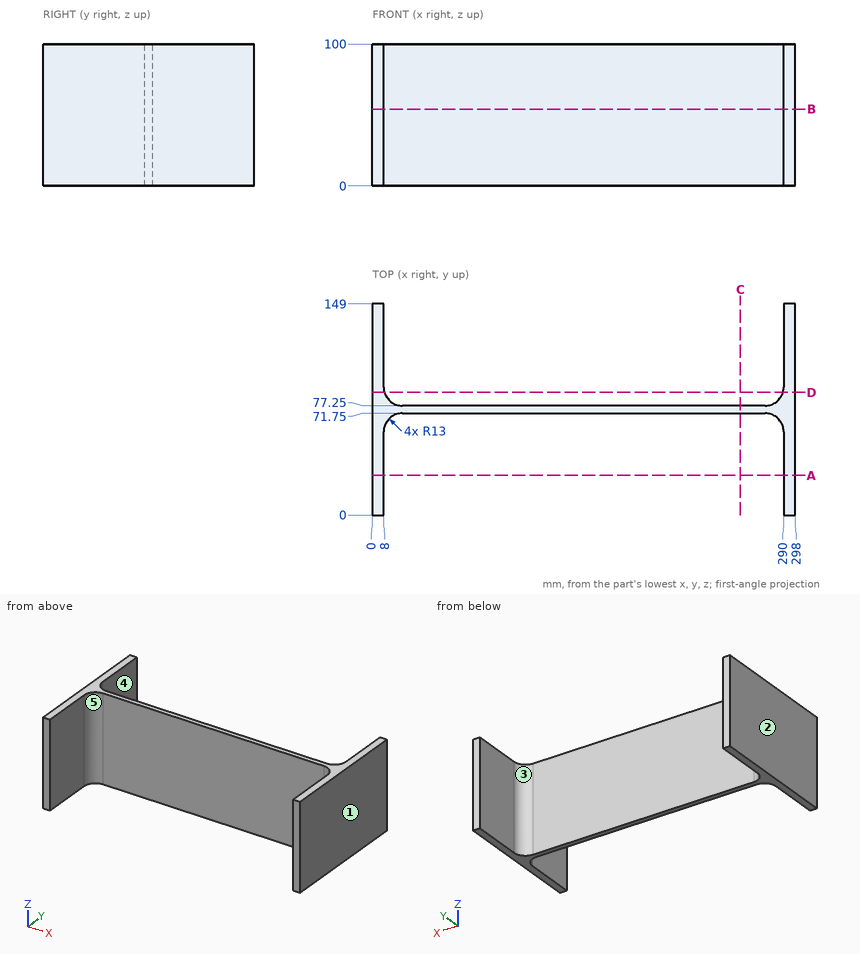
Can you work these out from the drawing? Everything is in mm from the part's minimum corner. A direction names the side the tool comes from. Give positions to 0.01 mm unless a question says otherwise; leave off trailing zeros. Order: outer loops, then holes, each group sorted by start corner. A loop starts at its lowest first (then second) coordinate and runs counter-clockwise, first axis right, second up. Notation, with made-up numbers: M 60.5,8.25 L 67.5,8.25 A17 ccw 67.5,30.25 Z; hole C 27,-3.75 d9. An arc over 180 degrees is marked long. Use a Markdown table: item, result. Add a question column.
Item 1: Suppose I cut it at A-A (y = 28). List the corners of the cut face in (x, z) for me.
Item 2: If I drill on L1, parallel to X at y = 108.5, z = 55.5; L2, parallel to Y at x = 226, z = 21; L3, parallel to X at y = 62, z = 65, over which ranges is the centre line in solid material (lowest first)? Write a range as [from, to].
Item 3: For the marked faces 4 and 5, which set-ups out of +Z, -Z, +X, -X, +Y, -Y let a thin tool reach every point of the face, with its end or its side?
Item 4: Suppose I cut it at D-D (y = 86.5). List the corners of the cut face in (x, z) for me.
Item 5: Suppose I cut it at C-C (x = 259.5). List the corners of the cut face in (y, z) for me.
Item 6: We'd pull the mould along X, two halves only. Please class the marked faces 1, 2 and 3: +X half, -X half, draft (parallel to the pull), parting line (faces both ways), or undercut.
Item 7: Will these pins go through, and if not, where does the flat tip stop? pin 1 (3 mm diameter, centred on x = 76.5, y = 70.5, fed in from +Z); pin 2 (4 mm diameter, centred on x = 246, z = 50.5, fed in from -Y); pin 3 (1 mm diameter, centred on x = 102.5, z = 56, fed in from +Y).
Item 8: Suppose I cut it at B-B (z = 54). List the corners of the cut face in (x, y) for me.
Answer sheet:
| question | item | result |
|---|---|---|
| 1 | outline | M 0,0 L 8,0 L 8,100 L 0,100 Z; M 290,0 L 298,0 L 298,100 L 290,100 Z |
| 2 | L1 | x = [0, 8], [290, 298] |
| 2 | L2 | y = [71.75, 77.25] |
| 2 | L3 | x = [0, 8.41], [289.59, 298] |
| 3 | face 4 | +Z, -Z, +Y |
| 3 | face 5 | +Z, -Z, -Y |
| 4 | outline | M 0,0 L 8.55,0 L 8.55,100 L 0,100 Z; M 289.45,0 L 298,0 L 298,100 L 289.45,100 Z |
| 5 | outline | M 71.75,0 L 77.25,0 L 77.25,100 L 71.75,100 Z |
| 6 | face 1 | +X half |
| 6 | face 2 | -X half |
| 6 | face 3 | undercut |
| 7 | pin 1 | stops at z = 100 |
| 7 | pin 2 | stops at y = 71.75 |
| 7 | pin 3 | stops at y = 77.25 |
| 8 | outline | M 0,0 L 8,0 L 8,58.75 A13 cw 21,71.75 L 277,71.75 A13 cw 290,58.75 L 290,0 L 298,0 L 298,149 L 290,149 L 290,90.25 A13 cw 277,77.25 L 21,77.25 A13 cw 8,90.25 L 8,149 L 0,149 Z |
